For this review, take the finished solid that the model builds, in its own axes (mm). Face numbers are marked on the shaded views. A direction names the side the tool comes from. Coordinates: 2 decimals unless noted, no trailing zeros. Order: outer loops, then holes, each group sorted by start corner. A loop starts at its lowest first (then second) coordinate and runs counter-clockwise, first axis right, second up. Notation, with made-up numbers: (22.5, 47.5) -> (78.5, 47.5) arc R27 cw to (78.5, 77.5) -> close; hole circle Ø7 at (-11.5, 32). An arc over 180 degrees is marked (long way). Answer as a JSON object with one key per item and string values. Group by question number.
1) Machinability: for the marked faces 4 and 5, which of the approach directions +Z, -Z, +X, -X, +Y, -Y give a long, thin tool a straight path to every point of the face, cutting with its end or side? Answer none if there is none.
2) Add section A-A, the plane y = -7.5. Write out the cut boundary in (x, z).
3) Add section B-B, the plane z = 16. Write out the cut boundary in (x, y), then the cut area to 3 significant figures.
4) Add section C-C, the plane y = -3.75. Write out the cut boundary in (x, z), then the cut area to 3 significant figures.
5) For pin 1 (4 mm diameter, centred on x = -1, y = -2.5, fed in from +Z), flat-tipped, find the tip position at first contact; note if it passes through.
6) Wall thickness on L1, parallel to Y at x = -3.5, z = 17.25; L2, parallel to X at y = 5, z = 16.6; L3, parallel to Y at x = -5.5, z = 16: over which ranges is each line inside the solid? List them lowest first.
7) Draft analysis for pull direction Y (two halves, no side actions). For the marked faces 1, 2 and 3, state which applies: +Y half, -Y half, draft (parallel to the pull), parting line (faces both ways), or undercut.
8) Add section D-D, the plane x = -7.5. Write out the cut boundary in (y, z), then the cut area to 3 significant figures.
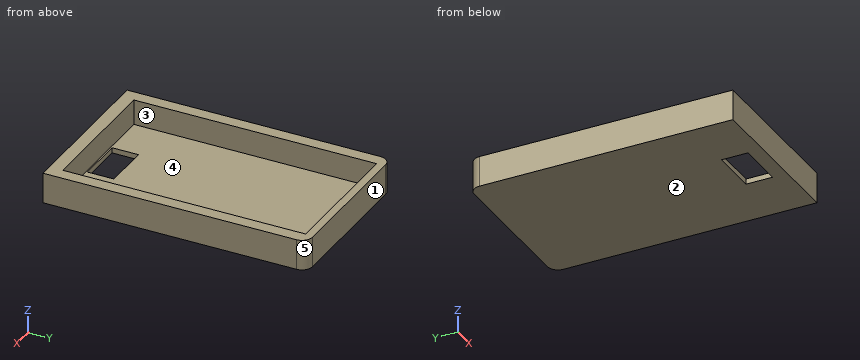
from build123d import *

# Parameters (mm, degrees)
ESQUISSE1_W        = 12.3
ESQUISSE1_H        = 19.9
ESQUISSE1_W_2      = 10.4
ESQUISSE1_H_2      = 18.3
BOSS_EXTRU_1_DEPTH = 2.3
ESQUISSE2_W        = 10.4
ESQUISSE2_H        = 18.3
ESQUISSE2_W_2      = 3.6
ESQUISSE2_H_2      = 2
BOSS_EXTRU_2_DEPTH = 0.4
CONG_1_R           = 0.8


with BuildPart() as part:
    # Esquisse1 → Boss.-Extru.1 (new body)
    with BuildSketch(Plane.XY.offset(18.1106)):
        with Locations((-3.99919357, -0.046839395)):
            Rectangle(ESQUISSE1_W, ESQUISSE1_H)
        with Locations((-3.99919357, 0.153160605)):
            Rectangle(ESQUISSE1_W_2, ESQUISSE1_H_2, mode=Mode.SUBTRACT)
    extrude(amount=-BOSS_EXTRU_1_DEPTH)

    # Esquisse2 → Boss.-Extru.2 (add)
    with BuildSketch(Plane(origin=(0, 0, 15.8106), x_dir=(-1, 0, 0), z_dir=(0, 0, -1))):
        with Locations((3.99919357, 0.153160605)):
            Rectangle(ESQUISSE2_W, ESQUISSE2_H)
        with Locations((3.99919357, -7.896839395)):
            Rectangle(ESQUISSE2_W_2, ESQUISSE2_H_2, mode=Mode.SUBTRACT)
    extrude(amount=-BOSS_EXTRU_2_DEPTH)

    # Congé1
    cong_1_edges = [part.edges().sort_by_distance(p)[0] for p in [
        (-10.14919357, 9.903160605, 16.9606),
        (2.15080643, 9.903160605, 16.9606),
    ]]
    fillet(cong_1_edges, radius=CONG_1_R)


solid = part.part
Output values:
{
 "1": {"face 4": "+Z", "face 5": "+Z, -Z, +X, +Y"},
 "2": {"outline": "(-10.15, 15.81) -> (-5.8, 15.81) -> (-5.8, 16.21) -> (-9.2, 16.21) -> (-9.2, 18.11) -> (-10.15, 18.11) -> close; (-2.2, 15.81) -> (2.15, 15.81) -> (2.15, 18.11) -> (1.2, 18.11) -> (1.2, 16.21) -> (-2.2, 16.21) -> close"},
 "3": {"outline": "(-10.15, -10) -> (2.15, -10) -> (2.15, 9.1) arc R0.8 ccw to (1.35, 9.9) -> (-9.35, 9.9) arc R0.8 ccw to (-10.15, 9.1) -> close; hole (-5.8, -8.9) -> (-2.2, -8.9) -> (-2.2, -6.9) -> (-5.8, -6.9) -> close", "area": "237 mm²"},
 "4": {"outline": "(-10.15, 15.81) -> (2.15, 15.81) -> (2.15, 18.11) -> (1.2, 18.11) -> (1.2, 16.21) -> (-9.2, 16.21) -> (-9.2, 18.11) -> (-10.15, 18.11) -> close", "area": "8.53 mm²"},
 "5": {"pin 1": "stops at z = 16.21"},
 "6": {"L1": "y = -10 to -9, 9.3 to 9.9", "L2": "x = -10.15 to -9.2, 1.2 to 2.15", "L3": "y = -10 to -8.9, -6.9 to 9.9"},
 "7": {"face 1": "+Y half", "face 2": "draft", "face 3": "undercut"},
 "8": {"outline": "(-10, 15.81) -> (9.9, 15.81) -> (9.9, 18.11) -> (9.3, 18.11) -> (9.3, 16.21) -> (-9, 16.21) -> (-9, 18.11) -> (-10, 18.11) -> close", "area": "11.0 mm²"}
}
